```python
from build123d import *

# Parameters (mm, degrees)
EXTRUDE_1_DEPTH     = 2.4
SKETCH_2_R          = 2.75
EXTRUDE_2_DEPTH     = 1.5
SKETCH_3_R          = 1.5
CUT_EXTRUDE_1_DEPTH = 6.732000814
FILLET_1_R          = 0.5


with BuildPart() as part:
    # 草图1 → 凸台-拉伸1 (new body)
    with BuildSketch(Plane(origin=(0, 0, 0), x_dir=(1, 0, 0), z_dir=(0, 1, 0))):
        Polygon((3.175426481, 0), (1.58771324, 2.75), (-1.58771324, 2.75), (-3.175426481, 0), (-1.58771324, -2.75), (1.58771324, -2.75), align=None)
    extrude(amount=EXTRUDE_1_DEPTH)

    # 草图2 → 凸台-拉伸2 (add)
    with BuildSketch(Plane(origin=(0, 2.4, 0), x_dir=(1, 0, 0), z_dir=(0, 1, 0))):
        with Locations(Location((0, 0, 0), (0, 0, 270))):
            Circle(SKETCH_2_R)
    extrude(amount=EXTRUDE_2_DEPTH)

    # 草图3 → 切除-拉伸1 (cut, through all)
    with BuildSketch(Plane(origin=(0, 3.9, 0), x_dir=(1, 0, 0), z_dir=(0, 1, 0))):
        with Locations(Location((0, 0, 0), (0, 0, 270))):
            Circle(SKETCH_3_R)
    extrude(amount=-CUT_EXTRUDE_1_DEPTH, mode=Mode.SUBTRACT)

    # 圆角1
    fillet_1_edges = [part.edges().sort_by_distance(p)[0] for p in [
        (0, 3.9, -2.75),
    ]]
    fillet(fillet_1_edges, radius=FILLET_1_R)


solid = part.part
```
Here's how the part is built. I have some questions about the finished solid (model axes, mm). A direction names the side the tool comes from. Give positions to 0.01 mm unless a question says otherwise; leave off trailing zeros. Loops run counter-clockwise (first coordinate to the right, second up) from the corner with the lowest first, then second, coordinate; pieces in that order, holes last. Notation, with made-up numbers: M 22,-12 L 64,-12 A25 ccw 64,16 Z; hole C 78,86.5 d1. An arc over 180 degrees is marked long. Use one line per item in the form item = value. Start each with the question number.
Q1. I need wall thicknesses on line 1 along X through (y, z) = (2.6, 0); line 2 along X through (y, z) = (2.05, -0.95); line 3 along Z through (x, y) = (-1, 1.2). Which ranges of each line are inside material? Lowest first, please.
Q2. If we section it at A-A (y = 2.3): Write out the boundary of the cut face in (x, z).
Q3. If we section it at B-B (y = 2.85): Write out the boundary of the cut face in (x, z).
Q4. Thinking about a two-plate mould opening in X: for faces 1 (the cylindrical face through (-2.685, 2.893, -0.596)), 2 (the flat face through (-2.37, 1.183, -1.394)), 3 (the cylindrical face through (0.45, 1.98, 1.43)), which applies, +X half, -X half, draft (parallel to the pull), parting line (faces both ways), or undercut?
Q5. Which directions (+Z, -Z, +X, -X, +Y, -Y) give clear straight access to the entire face, cutting with the end or side of a thin tool? Please do faces 4 (the flat face through (-1.5, 2.4, -2.5)), 5 (the flat face through (1.45, 2.4, 2.52)), 6 (the flat face through (-1.5, 2.4, 2.5)), 7 (the flat face through (1.45, 2.4, -2.52)).
Taken from the geometry:
q1.line_1 = -2.75 to -1.5, 1.5 to 2.75
q1.line_2 = -2.63 to -1.16, 1.16 to 2.63
q1.line_3 = -2.75 to -1.12, 1.12 to 2.75
q2.outline = M -3.18,0 L -1.59,-2.75 L 1.59,-2.75 L 3.18,0 L 1.59,2.75 L -1.59,2.75 Z; hole C 0,0 d3
q3.outline = C 0,0 d5.5; hole C 0,0 d3
q4.face_1 = parting line
q4.face_2 = -X half
q4.face_3 = undercut
q5.face_4 = -Z, -X, +Y
q5.face_5 = +Z, +X, +Y
q5.face_6 = +Z, -X, +Y
q5.face_7 = -Z, +X, +Y
